Check sheet for the drawn part. Datum: minimum x, y, z corner. Units: mm. A direction names the side the tool comes from. Give positions to 0.01 mm unless a question says otherwise; leave off trailing zeros. Loops run counter-clockwise (first coordinate to the right, second up) from the corner with the lowest first, then second, coordinate; pieces in that order, holes last. Notation, with made-up numbers: (12.25, 36.25) - (20.25, 36.25) arc R12 ccw to (20.25, 45.25) - close; hole circle Ø7 at (62.5, 8). An arc over 180 degrees is marked (long way). One line per item, written item: value. Start each with the question number.
1. Sectioned sample at A-A (z = 7). Record the cut outline in (x, y) (1 decimal).
2. Mould release check, pull along X, two halves, no side actions. Record for the marked faces 4, 5 and 6: pulls with the +X half, pulls with the -X half, needs draft (parallel to the pull), parting line crosses it, or undercut.
3. Access from +Z, -Z, +X, -X, +Y, -Y to the whole of each face (thin tool, end or side, straight path). Record for the marked faces 1, 2 and 3.
4. Scan lines: L1, parallel to X at y = 7.5, z = 6; L2, parallel to X at y = 13.5, z = 4.75; L3, parallel to Y at x = 56.5, z = 9.75. Record each from-to range of solid material in increasing order. Write a range as [from, to].
5. Sectioned sample at C-C (x = 55). Record the cut outline in (y, z), plus the area to 3 significant figures.
6. Sectioned sample at D-D (y = 48). Record the cut outline in (x, z), plus the area to 3 significant figures.
7. Gauge pin test, flat ends, axial feed: pin 1 (6 mm diameter, centred on y = 26.5, z = 6, fed in from -X); pin 2 (6 mm diameter, centred on y = 29.5, z = 8.5, fed in from -X); pin 3 (1.5 mm diameter, centred on y = 8.5, z = 3.5, fed in from +X); pin 4 (3 mm diameter, centred on x = 33.5, y = 33.5, fed in from -Z). Record the tip position at first contact, or that the pin passes through.
8. Sectioned sample at B-B (y = 31). Record the cut outline in (x, z) (1 decimal), plus the area to 4 significant figures.
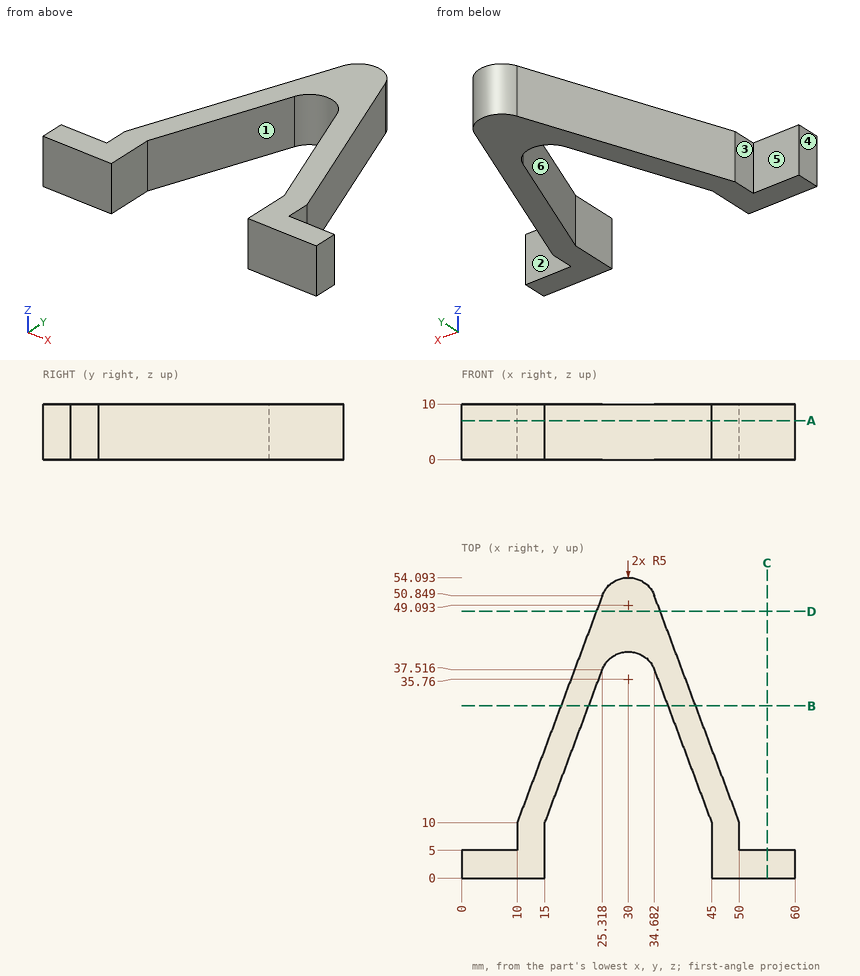
Results are:
1. outline: (0, 0) - (15, 0) - (15, 10) - (25.3, 37.5) arc R5 cw to (34.7, 37.5) - (45, 10) - (45, 0) - (60, 0) - (60, 5) - (50, 5) - (50, 10) - (34.7, 50.8) arc R5 ccw to (25.3, 50.8) - (10, 10) - (10, 5) - (0, 5) - close
2. face 4: pulls with the -X half
2. face 5: needs draft
2. face 6: undercut
3. face 1: +Z, -Z, -Y
3. face 2: +Z, -Z, +X, +Y
3. face 3: +Z, -Z, -X, +Y
4. L1: x = [10, 15], [45, 50]
4. L2: x = [11.31, 16.31], [43.69, 48.69]
4. L3: y = [0, 5]
5. outline: (0, 0) - (5, 0) - (5, 10) - (0, 10) - close
5. area: 50.0 mm^2
6. outline: (24.25, 0) - (35.75, 0) - (35.75, 10) - (24.25, 10) - close
6. area: 115 mm^2
7. pin 1: stops at x = 15.06
7. pin 2: stops at x = 16.19
7. pin 3: stops at x = 50
7. pin 4: passes through
8. outline: (17.9, 0) - (22.9, 0) - (22.9, 10) - (17.9, 10) - close; (37.1, 0) - (42.1, 0) - (42.1, 10) - (37.1, 10) - close
8. area: 100.0 mm^2
